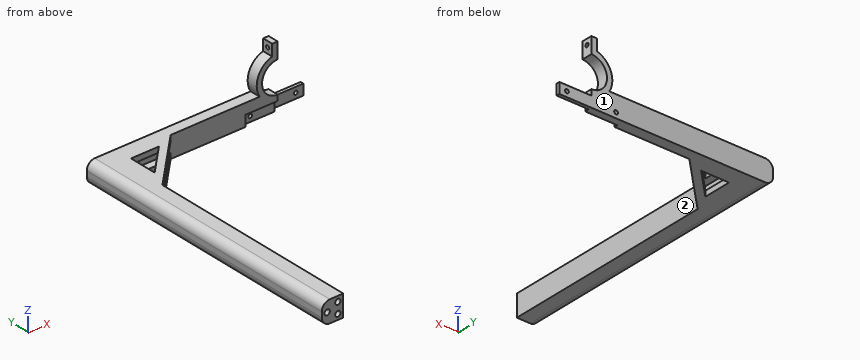
```python
from build123d import *

# Parameters (mm, degrees)
SKETCH1_W           = 20
SKETCH1_H           = 20
BOSS_EXTRUDE1_DEPTH = 260
SKETCH2_W           = 20
SKETCH2_H           = 10
BOSS_EXTRUDE2_DEPTH = 150
BOSS_EXTRUDE3_DEPTH = 10
CUT_EXTRUDE1_DEPTH  = 261
SKETCH4_R           = 1.75
CUT_EXTRUDE2_DEPTH  = 6
BOSS_EXTRUDE4_DEPTH = 5
FILLET3_R           = 7.5
SKETCH7_R           = 2.5
CUT_EXTRUDE3_DEPTH  = 8
SKETCH9_W           = 10
SKETCH9_H           = 3
BOSS_EXTRUDE6_DEPTH = 30
SKETCH10_W          = 10.1
SKETCH10_H          = 3.1
CUT_EXTRUDE4_DEPTH  = 30.2
SKETCH11_R          = 1.75
CUT_EXTRUDE5_DEPTH  = 261


with BuildPart() as part:
    # Sketch1 → Boss-Extrude1 (new body)
    with BuildSketch(Plane(origin=(0, 0, 0), x_dir=(1, 0, 0), z_dir=(0, 1, 0))):
        with Locations((10, 10)):
            Rectangle(SKETCH1_W, SKETCH1_H)
    extrude(amount=BOSS_EXTRUDE1_DEPTH)

    # Sketch2 → Boss-Extrude2 (add)
    with BuildSketch(Plane(origin=(20, 0, 0), x_dir=(0, 0, -1), z_dir=(1, 0, 0))):
        with Locations((10, 255)):
            Rectangle(SKETCH2_W, SKETCH2_H)
    extrude(amount=BOSS_EXTRUDE2_DEPTH)

    # Sketch3 → Boss-Extrude3 (add)
    with BuildSketch(Plane(origin=(0, 260, 0), x_dir=(1, 0, 0), z_dir=(0, 1, 0))):
        with BuildLine():
            Line((159.5, 0), (153.259330957, 0))
            ThreePointArc((153.259330957, 0), (151.938520085, -17.350710392), (165, -28.848076825))
            Line((165, -28.848076825), (165, -24.5))
            Line((165, -24.5), (170, -24.5))
            ThreePointArc((170, -24.5), (156.672397065, -15.711829829), (159.5, 0))
        make_face()
        with BuildLine():
            Line((165, -24.5), (165, -28.848076825))
            ThreePointArc((165, -28.848076825), (167.478839363, -29.336332358), (170, -29.5))
            Line((170, -29.5), (170, -24.5))
            Line((170, -24.5), (165, -24.5))
        make_face()
        with BuildLine():
            ThreePointArc((170, -29.5), (167.478839363, -29.336332358), (165, -28.848076825))
            Line((165, -28.848076825), (165, -39.5))
            Line((165, -39.5), (170, -39.5))
            Line((170, -39.5), (170, -29.5))
        make_face()
    extrude(amount=-BOSS_EXTRUDE3_DEPTH)

    # Sketch3<3> → Cut-Extrude1 (cut, through all)
    with BuildSketch(Plane(origin=(0, 260, 0), x_dir=(1, 0, 0), z_dir=(0, 1, 0))):
        with BuildLine():
            Line((170, 0), (170, 4.5))
            ThreePointArc((170, 4.5), (164.288170171, 3.327602935), (159.5, 0))
            Line((159.5, 0), (170, 0))
        make_face()
    extrude(amount=-CUT_EXTRUDE1_DEPTH, mode=Mode.SUBTRACT)

    # Sketch4 → Cut-Extrude2 (cut, through all)
    with BuildSketch(Plane.ZY.offset(-165)):
        with Locations((34.174038412, 255)):
            Circle(SKETCH4_R)
    extrude(amount=-CUT_EXTRUDE2_DEPTH, mode=Mode.SUBTRACT)

    # Sketch5 → Boss-Extrude4 (add)
    with BuildSketch(Plane.XY):
        Polygon((70, 250), (20, 200), (20, 250), align=None)
        Polygon((53.100505063, 243), (27, 216.899494937), (27, 243), align=None, mode=Mode.SUBTRACT)
    boss_extrude4 = extrude(amount=-BOSS_EXTRUDE4_DEPTH)

    # Mirror1: Boss-Extrude4 across plane
    add(boss_extrude4.mirror(Plane.XY.offset(-10)))

    # Fillet3
    fillet3_edges = [part.edges().sort_by_distance(p)[0] for p in [
        (0, 130, -20),
        (0, 130, 0),
    ]]
    fillet(fillet3_edges, radius=FILLET3_R)

    # Sketch7 → Cut-Extrude3 (cut)
    with BuildSketch(Plane.XZ):
        with Locations((15, -5)):
            Circle(SKETCH7_R)
        with Locations((5, -10)):
            Circle(SKETCH7_R)
        with Locations((15, -15)):
            Circle(SKETCH7_R)
    extrude(amount=-CUT_EXTRUDE3_DEPTH, mode=Mode.SUBTRACT)

    # Sketch9 → Boss-Extrude6 (add)
    with BuildSketch(Plane(origin=(170, 0, 0), x_dir=(0, 0, -1), z_dir=(1, 0, 0))):
        with Locations((15, 258.5)):
            Rectangle(SKETCH9_W, SKETCH9_H)
    extrude(amount=BOSS_EXTRUDE6_DEPTH)

    # Sketch10 → Cut-Extrude4 (cut)
    with BuildSketch(Plane(origin=(170, 0, 0), x_dir=(0, 0, -1), z_dir=(1, 0, 0))):
        with Locations((14.95, 251.55)):
            Rectangle(SKETCH10_W, SKETCH10_H)
    extrude(amount=-CUT_EXTRUDE4_DEPTH, mode=Mode.SUBTRACT)

    # Sketch11 → Cut-Extrude5 (cut, through all)
    with BuildSketch(Plane(origin=(0, 260, 0), x_dir=(1, 0, 0), z_dir=(0, 1, 0))):
        with Locations((147, 15)):
            Circle(SKETCH11_R)
    cut_extrude5 = extrude(amount=-CUT_EXTRUDE5_DEPTH, mode=Mode.SUBTRACT)

    # Mirror2: Cut-Extrude5 across plane
    add(cut_extrude5.mirror(Plane(origin=(170, 0, 0), x_dir=(0, 0, 1), z_dir=(1, 0, 0))), mode=Mode.SUBTRACT)


solid = part.part
```
Build history of the part. All positions in model axes, mm. Face numbers are marked on the shaded views. A direction names the side the tool comes from. Coordinates: 2 decimals unless noted, no trailing zeros. Order: outer loops, then holes, each group sorted by start corner. A loop starts at its lowest first (then second) coordinate and runs counter-clockwise, first axis right, second up. Notation, with made-up numbers: (28.25, 13.5) -> (33.25, 13.5) arc R21 ccw to (33.25, 40.5) -> close; hole circle Ø7 at (-30, 38). An arc over 180 degrees is marked (long way). Answer in a Markdown table with one row per item. Add a question column.
Q1. Band-saw the part on C-C, the plane z = 18.5. List the corners of the cut face in (x, y).
Q2. Band-saw the part on A-A, the plane x = 59. List the corners of the cut face in (y, z).
Q3. Band-saw the part on B-B, the plane x = 30.5. List the corners of the cut face in (y, z), then the cut area to 3 significant figures.
Q4. Band-saw the part on D-D, the plane x = 185.5. List the corners of the cut face in (y, z).
Q5. Wall check: line 1 along Z through (x, y) = (193, 257.75); line 2 along Z through (x, y) = (15, 2); line 3 along Y through (x, z) = (95.5, -6). Give the ranges that are in metal, low to high. Write a range as [from, to].
Q6. Which spindle directions (+Z, -Z, +X, -X, +Y, -Y) get a long thin tool onto all of the face, cutting with end or side? Do the marked faces 1 and 2. Say none if no direction does.
Q7. Drop flat-ended pins along their axis: pin 1 (4 mm diameter, centred on y = 230, z = -18, fed in from +X); pin 2 (3.5 mm diameter, centred on x = 184, y = 258, fed in from +Z); pin 3 (11 mm diameter, centred on x = 158.5, z = -17, fed in from -Y); pin 4 (5.5 mm diameter, centred on x = 15, z = -14, fed in from -Y). Give the stop position or say it passes through.
Answers follow:
| question | item | result |
|---|---|---|
| 1 | outline | (152.45, 250) -> (158.25, 250) -> (158.25, 260) -> (152.45, 260) -> close |
| 2 | outline | (239, -20) -> (260, -20) -> (260, 0) -> (239, 0) -> (239, -5) -> (250, -5) -> (250, -15) -> (239, -15) -> close |
| 3 | outline | (210.5, -20) -> (220.4, -20) -> (220.4, -15) -> (210.5, -15) -> close; (210.5, -5) -> (220.4, -5) -> (220.4, 0) -> (210.5, 0) -> close; (243, -20) -> (260, -20) -> (260, 0) -> (243, 0) -> (243, -5) -> (250, -5) -> (250, -15) -> (243, -15) -> close |
| 3 | area | 369 mm^2 |
| 4 | outline | (257, -20) -> (260, -20) -> (260, -10) -> (257, -10) -> close |
| 5 | line 1 | [-20, -16.75], [-13.25, -10] |
| 5 | line 2 | [-20, -17.5], [-12.5, -7.5], [-2.5, 0] |
| 5 | line 3 | [250, 260] |
| 6 | face 1 | +Z, -Z, +X, -X, +Y |
| 6 | face 2 | +X, -Y |
| 7 | pin 1 | x = 52 |
| 7 | pin 2 | z = -10 |
| 7 | pin 3 | y = 253.1 |
| 7 | pin 4 | y = 0 |
